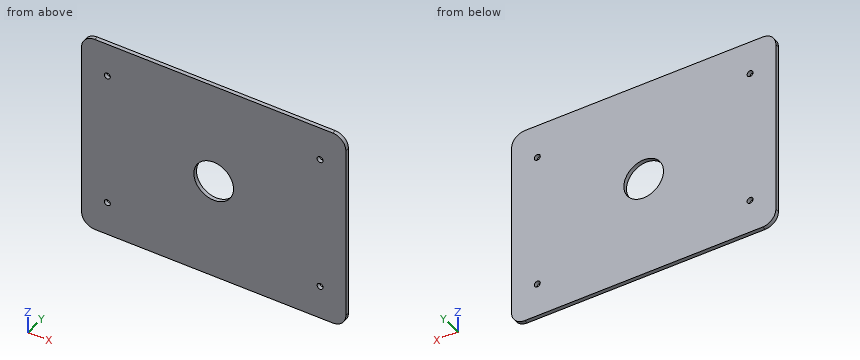
```python
from build123d import *

# Parameters (mm, degrees)
SKETCH1_W           = 200
SKETCH1_H           = 150
SKETCH1_R           = 2.25
SKETCH1_R_2         = 15
BOSS_EXTRUDE1_DEPTH = 3
FILLET1_R           = 10


with BuildPart() as part:
    # Sketch1 → Boss-Extrude1 (new body)
    with BuildSketch(Plane(origin=(0, 0, 0), x_dir=(1, 0, 0), z_dir=(0, 1, 0))):
        with Locations((45.2, -135.43)):
            Rectangle(SKETCH1_W, SKETCH1_H)
        with Locations((-35.3, -85.43)):
            Circle(SKETCH1_R, mode=Mode.SUBTRACT)
        with Locations((125.7, -85.43)):
            Circle(SKETCH1_R, mode=Mode.SUBTRACT)
        with Locations((125.7, -185.43)):
            Circle(SKETCH1_R, mode=Mode.SUBTRACT)
        with Locations((-35.3, -185.43)):
            Circle(SKETCH1_R, mode=Mode.SUBTRACT)
        with Locations((45.2, -135.43)):
            Circle(SKETCH1_R_2, mode=Mode.SUBTRACT)
    extrude(amount=BOSS_EXTRUDE1_DEPTH)

    # Fillet1
    fillet1_edges = [part.edges().sort_by_distance(p)[0] for p in [
        (145.2, 1.5, 210.43),
        (-54.8, 1.5, 210.43),
        (-54.8, 1.5, 60.43),
        (145.2, 1.5, 60.43),
    ]]
    fillet(fillet1_edges, radius=FILLET1_R)


solid = part.part
```
Geometry: final body of the model. Coordinates: model frame, mm. Round coordinates to 2 decimals unless told otherwise and drop trailing zeros. Order: outer loops, then holes, each group sorted by start corner. A loop starts at its lowest first (then second) coordinate and runs counter-clockwise, first axis right, second up. Notation, with made-up numbers: (2.5, 65.25) - (32.5, 65.25) arc R33 ccw to (32.5, 95.25) - close; hole circle Ø9 at (64.25, 27). An arc over 180 degrees is marked (long way). Write item = value, one per line. Start each with the question number.
Q1. Pin query (flat end, axial travel): pin 1 (4 mm diameter, centred on x = -35.3, z = 185.43, fed in from +Y). Return the tip coordinate at first contact, or that it passes through.
Q2. Ray query, line 1 (X direction, y = 2.15, z = 85.5); line 2 (Z direction, x = 125.7, y = 2.3); line 3 (X direction, y = 1.35, z = 184.5). Return the intervals inside material, ascending. Write a range as from..to.
Q3. Cut plane D-D on y = 2.3. Return the cut outline in (x, z), and give its area (3 significant figures).
Q4. Cut plane A-A on z = 135.43. Return the cut outline in (x, y).
Q5. Cut plane B-B on x = 125.7. Return the cut outline in (y, z).
Q6. Cut plane C-C on z = 85.43. Return the cut outline in (x, y).
Outcome:
q1.pin_1 = through
q2.line_1 = -54.8..-37.55, -33.05..123.45, 127.95..145.2
q2.line_2 = 60.43..83.18, 87.68..183.18, 187.68..210.43
q2.line_3 = -54.8..-37.35, -33.25..123.65, 127.75..145.2
q3.outline = (-54.8, 70.43) arc R10 ccw to (-44.8, 60.43) - (135.2, 60.43) arc R10 ccw to (145.2, 70.43) - (145.2, 200.43) arc R10 ccw to (135.2, 210.43) - (-44.8, 210.43) arc R10 ccw to (-54.8, 200.43) - close; hole circle Ø4.5 at (-35.3, 85.43); hole circle Ø4.5 at (-35.3, 185.43); hole circle Ø30 at (45.2, 135.43); hole circle Ø4.5 at (125.7, 85.43); hole circle Ø4.5 at (125.7, 185.43)
q3.area = 29,100 mm^2
q4.outline = (-54.8, 0) - (30.2, 0) - (30.2, 3) - (-54.8, 3) - close; (60.2, 0) - (145.2, 0) - (145.2, 3) - (60.2, 3) - close
q5.outline = (0, 60.43) - (3, 60.43) - (3, 83.18) - (0, 83.18) - close; (0, 87.68) - (3, 87.68) - (3, 183.18) - (0, 183.18) - close; (0, 187.68) - (3, 187.68) - (3, 210.43) - (0, 210.43) - close
q6.outline = (-54.8, 0) - (-37.55, 0) - (-37.55, 3) - (-54.8, 3) - close; (-33.05, 0) - (123.45, 0) - (123.45, 3) - (-33.05, 3) - close; (127.95, 0) - (145.2, 0) - (145.2, 3) - (127.95, 3) - close
